```python
from build123d import *

# Parameters (mm, degrees)
SKETCH1_W           = 8.784371834
SKETCH1_H           = 3.000075643
BOSS_EXTRUDE1_DEPTH = 3.175


with BuildPart() as part:
    # Sketch1 → Boss-Extrude1 (new body)
    with BuildSketch(Plane(origin=(0, 0, 0), x_dir=(1, 0, 0), z_dir=(0, 1, 0))):
        with BuildLine():
            Line((-9.483120155, -21.470892841), (-9.483120155, -25.850971148))
            Line((-9.483120155, -25.850971148), (-7.240182549, -25.850971148))
            Line((-7.240182549, -25.850971148), (-7.240182549, -22.850827141))
            Line((-7.240182549, -22.850827141), (-5.742820851, -22.850827141))
            Line((-5.742820851, -22.850827141), (-5.742820851, -25.850971148))
            Line((-5.742820851, -25.850971148), (-3.493751351, -25.850971148))
            Line((-3.493751351, -25.850971148), (-3.493751351, -22.850827141))
            Line((-3.493751351, -22.850827141), (-1.497298333, -22.850827141))
            Line((-1.497298333, -22.850827141), (-1.497298333, -18.850679894))
            Line((-1.497298333, -18.850679894), (-2.745036382, -18.850679894))
            Line((-2.745036382, -18.850679894), (-2.745036382, -18.750702276))
            Line((-2.745036382, -18.750702276), (-2.745036382, -16.250563552))
            Line((-2.745036382, -16.250563552), (-1.497298333, -16.250563552))
            Line((-1.497298333, -16.250563552), (-1.497298333, -12.750414262))
            Line((-1.497298333, -12.750414262), (1.49723009, -12.750414262))
            Line((1.49723009, -12.750414262), (1.49723009, -16.250563552))
            Line((1.49723009, -16.250563552), (2.745046129, -16.250563552))
            Line((2.745046129, -16.250563552), (2.745046129, -18.750702276))
            Line((2.745046129, -18.750702276), (2.745046129, -18.850679894))
            Line((2.745046129, -18.850679894), (1.49723009, -18.850679894))
            Line((1.49723009, -18.850679894), (1.49723009, -22.850827141))
            Line((1.49723009, -22.850827141), (5.190823665, -22.850827141))
            Line((5.190823665, -22.850827141), (5.190823665, -25.850971148))
            Line((5.190823665, -25.850971148), (9.483120155, -25.850971148))
            Line((9.483120155, -25.850971148), (9.483120155, 22.750856849))
            Line((9.483120155, 22.750856849), (6.488418889, 22.750856849))
            Line((6.488418889, 22.750856849), (6.488418889, 25.750995973))
            Line((6.488418889, 25.750995973), (3.493705241, 25.750995973))
            Line((3.493705241, 25.750995973), (3.493705241, 22.750856849))
            Line((3.493705241, 22.750856849), (1.497242474, 22.750856849))
            Line((1.497242474, 22.750856849), (1.497242474, 19.650735225))
            Line((1.497242474, 19.650735225), (2.745058512, 19.650735225))
            Line((2.745058512, 19.650735225), (2.745058512, 17.150659981))
            Line((2.745058512, 17.150659981), (1.497242474, 17.150659981))
            Line((1.497242474, 17.150659981), (1.497242474, 13.350397163))
            Line((1.497242474, 13.350397163), (-1.497285949, 13.350397163))
            Line((-1.497285949, 13.350397163), (-1.497285949, 17.150659981))
            Line((-1.497285949, 17.150659981), (-2.745023998, 17.150659981))
            Line((-2.745023998, 17.150659981), (-2.745023998, 19.650735225))
            Line((-2.745023998, 19.650735225), (-1.497285949, 19.650735225))
            Line((-1.497285949, 19.650735225), (-1.497285949, 22.750856849))
            Line((-1.497285949, 22.750856849), (-3.493751349, 22.750856849))
            Line((-3.493751349, 22.750856849), (-3.493751349, 25.750995973))
            Line((-3.493751349, 25.750995973), (-5.742820849, 25.750995973))
            Line((-5.742820849, 25.750995973), (-5.742820849, 22.750856849))
            Line((-5.742820849, 22.750856849), (-7.240182547, 22.750856849))
            Line((-7.240182547, 22.750856849), (-7.240182547, 25.750995973))
            Line((-7.240182547, 25.750995973), (-9.483120153, 25.750995973))
            Line((-9.483120153, 25.750995973), (-9.483120153, 21.370917666))
            add(Edge.make_bspline(
                [(-4.952518186, 15.886251248), (-5.015201934, 21.274211759), (-7.426547278, 21.343845481), (-9.483120153, 21.370917666)],
                knots=[6, 6, 6, 6, 7, 7, 7, 7], degree=3))
            add(Edge.make_bspline(
                [(-9.483120153, 9.692990904), (-7.240182547, 9.757380123), (-4.889844186, 10.498168659), (-4.952518186, 15.886251248)],
                knots=[5, 5, 5, 5, 6, 6, 6, 6], degree=3))
            Line((-9.483120153, 9.692990904), (-9.431179406, -8.834115587))
            add(Edge.make_bspline(
                [(-9.431179406, -8.834115587), (-7.188183308, -8.898499923), (-4.965366893, -9.64325846), (-4.995070997, -15.262909799)],
                knots=[1, 1, 1, 1, 2, 2, 2, 2], degree=3))
            add(Edge.make_bspline(
                [(-4.995070997, -15.262909799), (-5.024784848, -20.882307214), (-7.42654728, -21.443818214), (-9.483120155, -21.470892841)],
                knots=[2, 2, 2, 2, 3, 3, 3, 3], degree=3))
        make_face()
        with Locations((-0.598927132, -2.150035167)):
            Rectangle(SKETCH1_W, SKETCH1_H, mode=Mode.SUBTRACT)
    extrude(amount=BOSS_EXTRUDE1_DEPTH)


solid = part.part
```
Work out the finished part from the listing and answer in its coordinate system (mm). A direction names the side the tool comes from. Coordinates: 2 decimals unless noted, no trailing zeros. Write each loop counter-clockwise with the first axis right and the second up, starting at its lowest first coordinate (ties: lowest second). Pieces come first, ordered by that corner, then holes.
Q1. A cutting plane is placed at A-A, the plane x = -2.25. Give the vertices of the cut face in (y, z) (3 decimals), then the cut area to 3 significant figures.
Q2. Which of the six approach directions +Z, -Z, +X, -X, +Y, -Y give full straight-line access (tool end or side, diameter ignored) to faces 1 (the face through (-3.494, 2, 24)), 2 (the face through (0, 2, -13.35)), 3 (the face through (-2.745, 2, 18))?
Q3. A cutting plane is placed at B-B, the plane x = 7.25. Give the vertices of the cut face in (y, z) (3 decimals).
Q4. Find the intervals of material crossed by line 1 (Z direction, x = 2.5, y = 1.7); line 2 (Z direction, x = 0, y = 1.4); line 3 (Z direction, x = -7.5, y = 1.7), in increasing order.
Q5. Each of these flat-tipped pins is pushed along its axis until it touches: pin 1 Ø1.5 at (y, z) = (1.5, -24) entering from +X; pin 2 Ø8 at (x, z) = (4, -19) entering from -Y; pin 3 Ø0.6 at (x, y) = (-2, 2) entering from -Z; pin 4 Ø0.8 at (y, z) = (2, 17.5) entering from -X. Where does it stop, or does it pass through?
Q6. Determine the mould class of faces 4 (the face through (0, 3.175, 0)), 5 (the face through (2, 2, 16.251)) for opening direction X: released by +X, released by -X, zero draft, split by the parting line, or undercut.
Findings below:
1. outline: (0, -22.751) - (3.175, -22.751) - (3.175, -19.651) - (0, -19.651) - close; (0, -17.151) - (3.175, -17.151) - (3.175, 0.65) - (0, 0.65) - close; (0, 3.65) - (3.175, 3.65) - (3.175, 16.251) - (0, 16.251) - close; (0, 18.851) - (3.175, 18.851) - (3.175, 22.851) - (0, 22.851) - close
1. area: 119 mm2
2. face 1: +Z, +Y, -Y
2. face 2: -Z, +Y, -Y
2. face 3: +Y, -Y
3. outline: (0, -22.751) - (3.175, -22.751) - (3.175, 25.851) - (0, 25.851) - close
4. line 1: z = -22.75 to -19.65, -17.15 to 0.65, 3.65 to 16.25, 18.85 to 22.85
4. line 2: z = -13.35 to 0.65, 3.65 to 12.75
4. line 3: z = -25.75 to -21.16, -10.04 to 9.18, 21.14 to 25.85
5. pin 1: stops at x = 6.49
5. pin 2: stops at y = 0
5. pin 3: stops at z = -22.75
5. pin 4: stops at x = -5.24
6. face 4: zero draft
6. face 5: undercut
